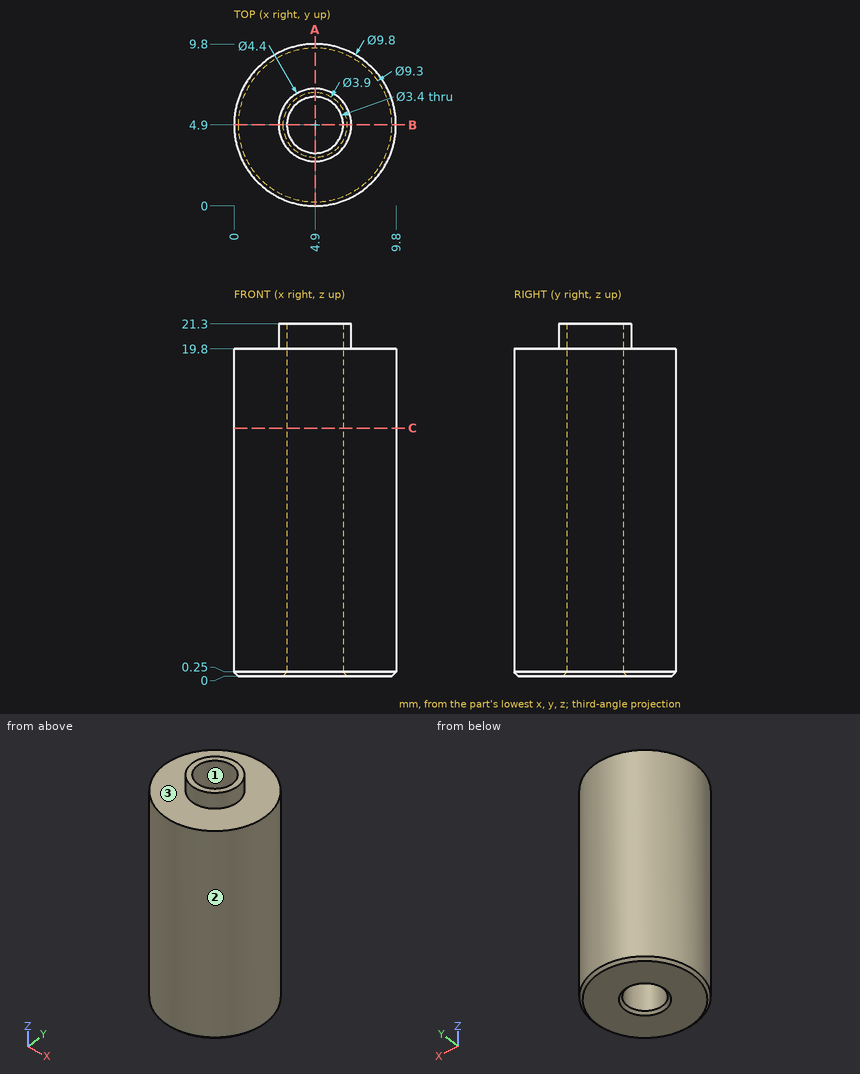
The figure shows three views and two pictorial views of one solid part (mm, origin at its lowest corner). Answer the questions. Round coordinates to 2 decimals unless told otherwise and drop trailing zeros. Write each loop counter-clockwise with the first axis right and the second up, starting at its lowest first coordinate (ties: lowest second). Pieces come first, ordered by that corner, then holes. Notation, with made-up numbers: (-8.5, -40) - (26.5, -40) arc R14 cw to (26.5, -32) - close; hole circle Ø10 at (38, 47.25). An arc over 180 degrees is marked (long way). Answer in a Markdown table with one row per item. Add a question column.
1. The mould has two halves that part along Y. Classify the marked faces 1, 2 and 3: +Y half, -Y half, draft (parallel to the pull), parting line (faces both ways), or undercut.
2. A cutting plane is placed at C-C, the plane z = 15. Determine the outline of the cut face in (x, y), and give its area (3 significant figures).
3. Find the intervals of material crossed by line 1 along Y through (x, z) = (4.9, 5.5); line 2 along Z through (x, y) = (1, 3.25); line 3 along Y through (x, z) = (6, 4.5), in increasing order. Write a range as from..to.
4. A cutting plane is placed at A-A, the plane x = 4.9. Determine the outline of the cut face in (y, z).
5. Given pin 1 (2 mm diameter, centred on y = 6.5, z = 16.5, fed in from +X); pin 2 (1 mm diameter, centred on x = 1.5, z = 8.5, fed in from +Y); pin 3 (4 mm diameter, centred on y = 2, z = 8.5, fed in from -X), each flat-ended and moving along its own axis, determine where each tip first touches the part or whether it passes through.
Worked out:
| question | item | result |
|---|---|---|
| 1 | face 1 | undercut |
| 1 | face 2 | parting line |
| 1 | face 3 | draft |
| 2 | outline | circle Ø9.8 at (4.9, 4.9); hole circle Ø3.4 at (4.9, 4.9) |
| 2 | area | 66.4 mm^2 |
| 3 | line 1 | 0..3.2, 6.6..9.8 |
| 3 | line 2 | 0..19.8 |
| 3 | line 3 | 0.13..3.6, 6.2..9.67 |
| 4 | outline | (0, 0.25) - (0.25, 0) - (2.95, 0) - (3.2, 0.25) - (3.2, 21.3) - (2.7, 21.3) - (2.7, 19.8) - (0, 19.8) - close; (6.6, 0.25) - (6.85, 0) - (9.55, 0) - (9.8, 0.25) - (9.8, 19.8) - (7.1, 19.8) - (7.1, 21.3) - (6.6, 21.3) - close |
| 5 | pin 1 | x = 9.76 |
| 5 | pin 2 | y = 8.85 |
| 5 | pin 3 | x = 0.08 |
